Design review of the part built by this model. Coordinates are the model's own, in mm. A direction names the side the tool comes from. Coordinates: 2 decimals unless noted, no trailing zeros. Write each loop counter-clockwise with the first axis right and the second up, starting at its lowest first coordinate (ties: lowest second). Pieces come first, ordered by that corner, then holes. Notation, with made-up numbers: (-27, 43.5) - (1, 43.5) arc R19 cw to (1, 74.5) - close; hole circle Ø5 at (56, 66.5). An arc over 180 degrees is marked (long way). Answer as CSV lines item,"result". Start each with the question number.
Q1. Clearance check with flat-ended pins moving along their axes: pin 1 (2 mm diameter, centred on x = -1.5, z = -6, fed in from -Y); pin 2 (12 mm diameter, centred on y = 0.5, z = 2.5, fed in from -X); pin 3 (3 mm diameter, centred on y = -5, z = 8.66, fed in from +X); pin 4 (4 mm diameter, centred on y = 9.5, z = -4, fed in from +X). State where each tip first meets the part, or that it passes through.
Q2. We need section D-D (x = -4). Write out the cut boundary in (y, z), plus the area to 3 significant figures.
Q3. We need section B-B (y = 0). Write out the cut boundary in (x, z), plus the area to 3 significant figures.
Q4. We need section A-A (z = 0). Write out the cut boundary in (x, y).
Q5. For line 1 along Z through (x, y) = (0.6, -5); line 2 along X through (y, z) = (8.5, -12.5); line 3 along Y through (x, z) = (4, 5), list the stretches that pass through material, from the lowest coordinate up. Write a range as [from, to].
Q6. We need section C-C (x = 3.25). Write out the cut boundary in (y, z), plus the area to 3 significant figures.
Q7. Machinability: for faces 1 (the face through (4.542, -4.444, -20.013)), 2 (the face through (0.021, 11.735, 0.228)), 3 (the face through (-2.01, -1.19, -5.37)), which of the approach directions +Z, -Z, +X, -X, +Y, -Y give a long, thin tool a straight path to every point of the face, cutting with its end or side? Answer none if there is none.
from build123d import *

# Parameters (mm, degrees)
SKETCH_2_R               = 1.75
CUT_EXTRUDE_1_DEPTH      = 8.5
CUT_EXTRUDE_1_DEPTH_BACK = 8.5


with BuildPart() as part:
    # ｽｹｯﾁ1 → 回転1 (revolve)
    with BuildSketch(Plane.XY):
        with BuildLine():
            Line((-2.5, 4.5), (2.5, 4.5))
            Line((2.5, 4.5), (2.5, 5.5))
            Line((2.5, 5.5), (1.5, 5.5))
            Line((1.5, 5.5), (1.5, 20.5))
            Line((1.5, 20.5), (7.5, 20.5))
            ThreePointArc((7.5, 20.5), (0, 28), (-7.5, 20.5))
            Line((-7.5, 20.5), (-1.5, 20.5))
            Line((-1.5, 20.5), (-1.5, 5.5))
            Line((-1.5, 5.5), (-2.5, 5.5))
            Line((-2.5, 5.5), (-2.5, 4.5))
        make_face()
    revolve(axis=Axis((0, 0, 0), (1, 0, 0)))

    # ｽｹｯﾁ2 → ｶｯﾄ - 押し出し1 (cut, two sides)
    with BuildSketch(Plane(origin=(0, 0, 0), x_dir=(0, 0, -1), z_dir=(1, 0, 0))) as cut_extrude_1_sk:
        with Locations((0, 10)):
            Circle(SKETCH_2_R)
        with Locations((8.660254038, -5)):
            Circle(SKETCH_2_R)
        with Locations((-8.660254038, -5)):
            Circle(SKETCH_2_R)
    extrude(amount=CUT_EXTRUDE_1_DEPTH, mode=Mode.SUBTRACT)
    extrude(cut_extrude_1_sk.sketch, amount=-CUT_EXTRUDE_1_DEPTH_BACK, mode=Mode.SUBTRACT)


solid = part.part
Results list:
1,pin 1,"stops at y = -27.46"
1,pin 2,"stops at x = -2.5"
1,pin 3,"passes through"
1,pin 4,"stops at x = 1.5"
2,outline,"circle Ø53.69 at (0, 0); hole circle Ø41 at (0, 0)"
2,area,"944 mm2"
3,outline,"(-7.5, -20.5) arc R7.5 ccw to (7.5, -20.5) - (1.5, -20.5) - (1.5, -5.5) - (2.5, -5.5) - (2.5, -4.5) - (-2.5, -4.5) - (-2.5, -5.5) - (-1.5, -5.5) - (-1.5, -20.5) - close; (-7.5, 20.5) - (-1.5, 20.5) - (-1.5, 5.5) - (-2.5, 5.5) - (-2.5, 4.5) - (2.5, 4.5) - (2.5, 5.5) - (1.5, 5.5) - (1.5, 20.5) - (7.5, 20.5) arc R7.5 ccw to start"
3,area,"277 mm2"
4,outline,"(-7.5, -20.5) arc R7.5 ccw to (7.5, -20.5) - (1.5, -20.5) - (1.5, -5.5) - (2.5, -5.5) - (2.5, -4.5) - (-2.5, -4.5) - (-2.5, -5.5) - (-1.5, -5.5) - (-1.5, -20.5) - close; (-7.5, 20.5) - (-1.5, 20.5) - (-1.5, 11.75) - (1.5, 11.75) - (1.5, 20.5) - (7.5, 20.5) arc R7.5 ccw to start; (-2.5, 4.5) - (2.5, 4.5) - (2.5, 5.5) - (1.5, 5.5) - (1.5, 8.25) - (-1.5, 8.25) - (-1.5, 5.5) - (-2.5, 5.5) - close"
5,line 1,"z = [-27.53, -10.41], [-6.91, 6.91], [10.41, 27.53]"
5,line 2,"x = [-1.5, 1.5]"
5,line 3,"y = [-26.37, -19.88], [19.88, 26.37]"
6,outline,"circle Ø54.52 at (0, 0); hole circle Ø41 at (0, 0)"
6,area,"1,010 mm2"
7,face 1,"+X"
7,face 2,"+X, -X"
7,face 3,"-X"
